Verification items for this drawing (mm, ordinates from the low corner). Round coordinates to 2 decimals unless told otherwise and drop trailing zeros. Order: outer loops, then holes, each group sorted by start corner. A loop starts at its lowest first (then second) coordinate and runs counter-clockwise, first axis right, second up. Notation, with made-up numbers: (81.25, 68.25) -> (134.25, 68.25) arc R20 cw to (134.25, 87.25) -> close; hole circle Ø5 at (63, 78). An arc over 180 degrees is marked (long way). Answer in a Markdown table with one row per item. Add a question column.
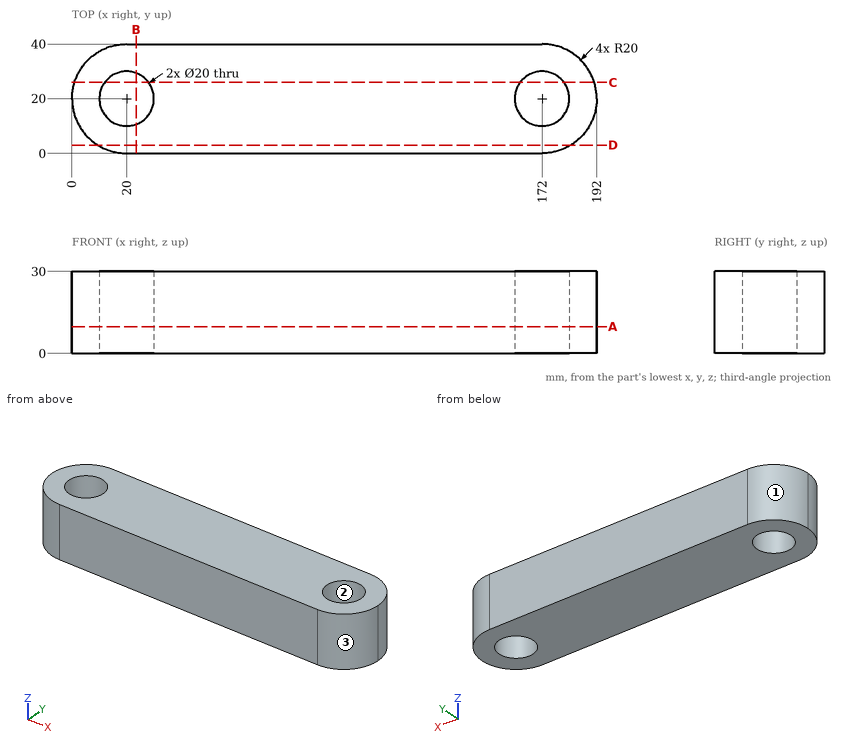
1) Depth check by flat-ended pin: P1, Ø18, axis at x = 172, y = 20, coming from the -Z side; P2, Ø2, axis at y = 26, z = 17, coming from the +X side (3 decimals); P3, Ø1.5, axis at y = 23.5, z = 15, coming from the +X side; P4, Ø2, axis at y = 28, z = 23, coming from the -X side (3 decimals). Enter the tip coordinate at first touch or a pass-through.
2) Thickness scan on L1, parallel to X at y = 16.5, z = 4.5; L2, parallel to Y at x = 20, z = 18.25; L3, parallel to X at y = 27, z = 2.75 (1 decimal). Record the ranges inside material, lowest first. Write a range as [from, to].
3) Draft check along X on the marked faces 1, 2 and 3. Enter one of: +X half, -X half, draft (parallel to the pull), parting line (faces both ways), or undercut.
4) Cross-section at A-A, the plane z = 9.75. Give the number of separate pieces and of enclosed holes in the cut face, and give its area (3 significant figures).
5) Cross-section at B-B, the plane x = 23.5. Record the boundary of the cut face in (y, z), and give its area (3 significant figures).
6) Cross-section at C-C, the plane y = 26. Record the boundary of the cut face in (x, z).
7) Cross-section at D-D, the plane y = 3. Record the boundary of the cut face in (x, z), and give its area (3 significant figures).
Results below:
| question | item | result |
|---|---|---|
| 1 | P1 | through |
| 1 | P2 | x = 191.365 |
| 1 | P3 | x = 191.81 |
| 1 | P4 | x = 1.265 |
| 2 | L1 | [0.31, 10.63], [29.37, 162.63], [181.37, 191.69] |
| 2 | L2 | [0, 10], [30, 40] |
| 2 | L3 | [1.3, 12.9], [27.1, 164.9], [179.1, 190.7] |
| 3 | face 1 | -X half |
| 3 | face 2 | undercut |
| 3 | face 3 | +X half |
| 4 | separate pieces | 1 |
| 4 | enclosed holes | 2 |
| 4 | area | 6,710 mm² |
| 5 | outline | (0, 0) -> (10.63, 0) -> (10.63, 30) -> (0, 30) -> close; (29.37, 0) -> (40, 0) -> (40, 30) -> (29.37, 30) -> close |
| 5 | area | 638 mm² |
| 6 | outline | (0.92, 0) -> (12, 0) -> (12, 30) -> (0.92, 30) -> close; (28, 0) -> (164, 0) -> (164, 30) -> (28, 30) -> close; (180, 0) -> (191.08, 0) -> (191.08, 30) -> (180, 30) -> close |
| 7 | outline | (9.46, 0) -> (182.54, 0) -> (182.54, 30) -> (9.46, 30) -> close |
| 7 | area | 5,190 mm² |
